```python
from build123d import *

# Parameters (mm, degrees)
BOSS_EXTRUDE1_DEPTH = 2.54
BOSS_EXTRUDE2_DEPTH = 2.54


with BuildPart() as part:
    # Sketch1 → Boss-Extrude1 (new body)
    with BuildSketch(Plane(origin=(0, -403.215393304, 914.186019304), x_dir=(1, 0, 0), z_dir=(0, -0.403554778, 0.914955486))):
        with BuildLine():
            Line((41.090457211, 1205.302750155), (41.090457211, 1181.172750155))
            add(Edge.make_bspline(
                [(41.090457211, 1181.172750155), (41.090457211, 1179.500406586), (40.786106444, 1177.855480514), (40.627250629, 1176.996911717), (40.38674257, 1176.156490093), (40.140401941, 1175.295687376), (39.810465838, 1174.462215303), (39.474066056, 1173.612414933), (39.053823577, 1172.79959973), (38.627425101, 1171.974877856), (38.118810853, 1171.196866161), (37.605369582, 1170.411470717), (37.013273567, 1169.682127132), (36.418695318, 1168.949725934), (35.750879918, 1168.281870238), (35.083841269, 1167.614791339), (34.350623023, 1167.019476589), (33.622163357, 1166.428025426), (32.835883994, 1165.913939303), (32.058807597, 1165.405870274), (31.233150426, 1164.978926578), (30.421305456, 1164.559125111), (29.570534852, 1164.222284318), (28.738051446, 1163.892683872), (27.876260062, 1163.646007586), (27.036829788, 1163.40573187), (26.177269641, 1163.246643712), (24.532849383, 1162.942292945), (22.86, 1162.942292945)],
                knots=[0, 0, 0, 0.125, 0.125, 0.1875, 0.1875, 0.25, 0.25, 0.3125, 0.3125, 0.375, 0.375, 0.4375, 0.4375, 0.5, 0.5, 0.5625, 0.5625, 0.625, 0.625, 0.6875, 0.6875, 0.75, 0.75, 0.8125, 0.8125, 0.875, 0.875, 1, 1, 1], degree=2))
            ThreePointArc((22.86, 1162.942292945), (17.107545571, 1156.658209277), (15.02386871, 1148.397535561))
            ThreePointArc((15.02386871, 1148.397535561), (0, 1133.373666883), (-15.02386871, 1148.397535561))
            ThreePointArc((-15.02386871, 1148.397535561), (-17.107545571, 1156.658209277), (-22.86, 1162.942292945))
            add(Edge.make_bspline(
                [(-41.090457211, 1181.172750155), (-41.090457211, 1179.500406586), (-40.786106444, 1177.855480514), (-40.627250629, 1176.996911717), (-40.38674257, 1176.156490093), (-40.140401941, 1175.295687376), (-39.810465838, 1174.462215303), (-39.474066056, 1173.612414933), (-39.053823577, 1172.79959973), (-38.627425101, 1171.974877856), (-38.118810853, 1171.196866161), (-37.605369582, 1170.411470717), (-37.013273567, 1169.682127132), (-36.418695318, 1168.949725934), (-35.750879918, 1168.281870238), (-35.083841269, 1167.614791339), (-34.350623023, 1167.019476589), (-33.622163357, 1166.428025426), (-32.835883994, 1165.913939303), (-32.058807597, 1165.405870274), (-31.233150426, 1164.978926578), (-30.421305456, 1164.559125111), (-29.570534852, 1164.222284318), (-28.738051446, 1163.892683872), (-27.876260062, 1163.646007586), (-27.036829788, 1163.40573187), (-26.177269641, 1163.246643712), (-24.532849383, 1162.942292945), (-22.86, 1162.942292945)],
                knots=[0, 0, 0, 0.125, 0.125, 0.1875, 0.1875, 0.25, 0.25, 0.3125, 0.3125, 0.375, 0.375, 0.4375, 0.4375, 0.5, 0.5, 0.5625, 0.5625, 0.625, 0.625, 0.6875, 0.6875, 0.75, 0.75, 0.8125, 0.8125, 0.875, 0.875, 1, 1, 1], degree=2))
            Line((-41.090457211, 1181.172750155), (-41.090457211, 1205.302750155))
            ThreePointArc((-41.090457211, 1205.302750155), (-39.838195765, 1213.399088759), (-34.922129755, 1219.952801638))
            Line((-34.922129755, 1219.952801638), (-124.282704843, 1219.952801638))
            ThreePointArc((-124.282704843, 1219.952801638), (-133.452528355, 1219.261665344), (-142.415163066, 1217.203872436))
            Line((-142.415163066, 1217.203872436), (-11.602437283, 1107.542547866))
            ThreePointArc((-11.602437283, 1107.542547866), (0, 1110.539391573), (11.602437283, 1107.542547866))
            Line((11.602437283, 1107.542547866), (142.415163066, 1217.203872436))
            ThreePointArc((142.415163066, 1217.203872436), (133.452528355, 1219.261665344), (124.282704843, 1219.952801638))
            Line((124.282704843, 1219.952801638), (34.922129755, 1219.952801638))
            ThreePointArc((34.922129755, 1219.952801638), (39.838195765, 1213.399088759), (41.090457211, 1205.302750155))
        make_face()
    boss_extrude1 = extrude(amount=BOSS_EXTRUDE1_DEPTH)


with BuildPart() as body_2:
    # Sketch2 → Boss-Extrude2 (new body)
    with BuildSketch(Plane(origin=(250.456709511, -189.811186969, 1179.622087881), x_dir=(-0.978727634, -0.032622557, 0.202553664), z_dir=(-0.205163879, 0.155485551, -0.966298104))):
        with BuildLine():
            Line((438.824397172, 866.073971669), (451.606917208, 795.421913218))
            ThreePointArc((451.606917208, 795.421913218), (450.542773626, 791.265264069), (446.699876764, 789.356788913))
            Line((446.699876764, 789.356788913), (277.752918196, 780.24161181))
            ThreePointArc((277.752918196, 780.24161181), (281.389861334, 801.904197312), (267.155321643, 818.633597954))
            Line((267.155321643, 818.633597954), (400.876040527, 924.729024753))
            ThreePointArc((400.876040527, 924.729024753), (425.219058104, 898.875003324), (438.824397172, 866.073971669))
        make_face()
    boss_extrude2 = extrude(amount=BOSS_EXTRUDE2_DEPTH)


with BuildPart() as part_1:
    add(part.part)

    add(body_2.part)  # Mirror7 merges body 2
    # Mirror7: Boss-Extrude1, Boss-Extrude2 across plane
    add(boss_extrude1.mirror(Plane(origin=(0, 0, 0), x_dir=(0, 0, 1), z_dir=(1, 0, 0))))
    add(boss_extrude2.mirror(Plane(origin=(0, 0, 0), x_dir=(0, 0, 1), z_dir=(1, 0, 0))))


solid = part_1.part
```
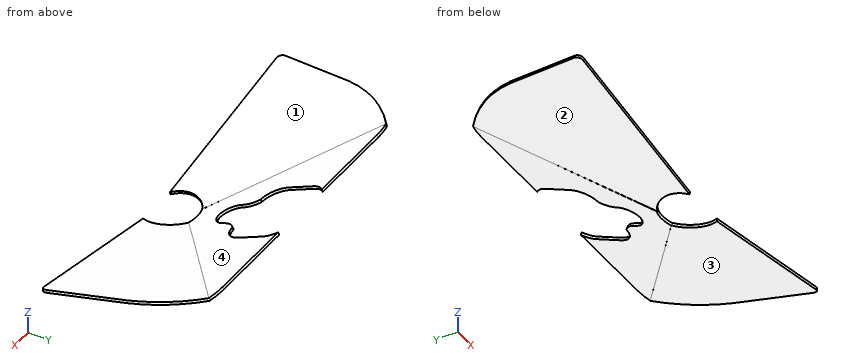
Source: CAD feature listing. Evaluate the final solid. Frame: model axes, mm. Face numbers are marked on the shaded views. A direction names the side the tool comes from. Give positions to 0.01 mm unless a question says otherwise; leave off trailing zeros. Order: outer loops, then holes, each group sorted by start corner. A loop starts at its lowest first (then second) coordinate and runs counter-clockwise, first axis right, second up.
(1) Pull-direction query (X, two-part tool) for the marked faces 1 and 2; classes: +X half, -X half, draft (parallel to the pull), parting line (faces both ways), or undercut.
(2) Access query for the marked faces 3 and 4. Directions: +Z, -Z, +X, -X, +Y, -Y. A direction counts if a zero-diameter tool reaches every point of the face in a straight line with its end or side. Return the directions, or none.
(3) Section query B-B (x = 112.5). Return the cut outline in (y, z), plus the area to 3 significant figures.
(4) Material intervals for line 1 along Z through (x, y) = (21, 608); line 2 along Z through (x, y) = (61, 632); line 3 along Y through (x, z) = (-61.5, 1384), sorted ascending.
(5) Contact query for flat-ended pins moving along their axis: P1, Ø6, axis at x = -133.5, z = 1381.5, coming from the -Y side; P2, Ø2, axis at x = 28.5, y = 638.5, coming from the -Z side; P3, Ø1.5, axis at x = 88.5, y = 653, coming from the +Z side; P4, Ø2, axis at x = -148, z = 1383, coming from the +Y side. Output: stop coordinate, or through.
Outcome:
1. face 1: undercut
1. face 2: -X half
2. face 3: -Z, +X, +Y
2. face 4: +Z, -Y
3. outline: (573.38, 1379.49) - (573.77, 1376.92) - (687.53, 1395.23) - (687.53, 1395.27) - (712.99, 1406.5) - (711.96, 1408.83) - (686.83, 1397.74) - close
3. area: 369 mm2
4. line 1: z = 1363 to 1365.63
4. line 2: z = 1375.36 to 1377.99
4. line 3: y = 655.67 to 661.97
5. P1: stops at y = 573.78
5. P2: stops at z = 1373.21
5. P3: stops at z = 1387.4
5. P4: passes through
